Verification items for the finished model (mm, model axes). Round coordinates to 2 decimals unless told otherwise and drop trailing zeros. Order: outer loops, then holes, each group sorted by start corner. A loop starts at its lowest first (then second) coordinate and runs counter-clockwise, first axis right, second up. Notation, with made-up numbers: M 78,46 L 128,46 A21 ccw 128,62 Z; hole C 57.25,79 d4. An arc over 180 degrees is marked long. Write item = value, one per line. Start each with the question number.
from build123d import *

# Parameters (mm, degrees)
SKETCH2_W           = 70
SKETCH2_H           = 45
BOSS_EXTRUDE1_DEPTH = 1.5
SKETCH3_R           = 1.625
SKETCH3_R_2         = 6
CUT_EXTRUDE1_DEPTH  = 2.5
CUT_EXTRUDE2_DEPTH  = 2.5


with BuildPart() as part:
    # Sketch2 → Boss-Extrude1 (new body)
    with BuildSketch(Plane(origin=(0, 0, 0), x_dir=(1, 0, 0), z_dir=(0, 1, 0))):
        Rectangle(SKETCH2_W, SKETCH2_H)
    extrude(amount=BOSS_EXTRUDE1_DEPTH)

    # Sketch3 → Cut-Extrude1 (cut, through all)
    with BuildSketch(Plane(origin=(0, 1.5, 0), x_dir=(1, 0, 0), z_dir=(0, 1, 0))):
        with Locations((-31, -18.5)):
            Circle(SKETCH3_R)
        with Locations((-31, 18.5)):
            Circle(SKETCH3_R)
        with Locations((31, 18.5)):
            Circle(SKETCH3_R)
        with Locations((31, -18.5)):
            Circle(SKETCH3_R)
        with Locations((-25, 0)):
            Circle(SKETCH3_R_2)
        with Locations((25, 0)):
            Circle(SKETCH3_R_2)
    extrude(amount=-CUT_EXTRUDE1_DEPTH, mode=Mode.SUBTRACT)

    # Sketch4 → Cut-Extrude2 (cut, through all)
    with BuildSketch(Plane(origin=(0, 1.5, 0), x_dir=(1, 0, 0), z_dir=(0, 1, 0))):
        Polygon((-10.6, -18), (-10.6, -15.4), (-15.75, -10.25), (-18, -10.25), (-18, 10.25), (-15.75, 10.25), (-8, 18), (12, 18), (12, 14), (18, 8), (18, -10.6), (15.4, -10.6), (8, -18), align=None)
    extrude(amount=-CUT_EXTRUDE2_DEPTH, mode=Mode.SUBTRACT)


solid = part.part
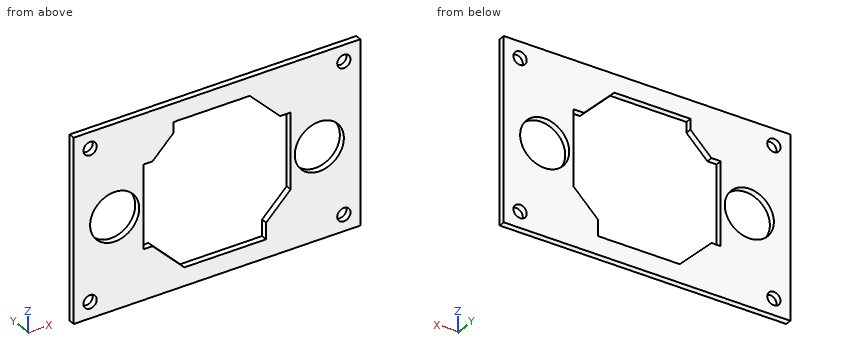
1) Scan lines: probe 1 along X at (y, z) = (0.7, 0); probe 2 along X at (y, z) = (0.3, 18.5) (3 decimals); probe 3 along Z at (x, y) = (-2, 1.35). Record each from-to range of solid material in increasing order.
2) Cross-section at A-A, the plane z = 9. Enter the section's corners in (x, y), then the cut area to 3 significant figures.
3) Cross-section at D-D, the plane y = 0.6. Enter the section's corners in (x, z) (3 decimals).
4) Cross-section at B-B, the plane x = -0.5. Enter the section's corners in (y, z).
5) Cross-section at C-C, the plane z = 0. Enter the section's corners in (x, y), then the cut area to 3 significant figures.
Geometry results:
q1.probe_1 = -35 to -31, -19 to -18, 18 to 19, 31 to 35
q1.probe_2 = -35 to -32.625, -29.375 to 29.375, 32.625 to 35
q1.probe_3 = -22.5 to -18, 18 to 22.5
q2.outline = M -35,0 L -18,0 L -18,1.5 L -35,1.5 Z; M 18,0 L 35,0 L 35,1.5 L 18,1.5 Z
q2.area = 51.0 mm^2
q3.outline = M -35,-22.5 L 35,-22.5 L 35,22.5 L -35,22.5 Z; hole C -31,-18.5 d3.25; hole C -31,18.5 d3.25; hole C -25,0 d12; hole M -18,-10.25 L -15.75,-10.25 L -8,-18 L 12,-18 L 12,-14 L 18,-8 L 18,10.6 L 15.4,10.6 L 8,18 L -10.6,18 L -10.6,15.4 L -15.75,10.25 L -18,10.25 Z; hole C 25,0 d12; hole C 31,-18.5 d3.25; hole C 31,18.5 d3.25
q4.outline = M 0,-22.5 L 1.5,-22.5 L 1.5,-18 L 0,-18 Z; M 0,18 L 1.5,18 L 1.5,22.5 L 0,22.5 Z
q5.outline = M -35,0 L -31,0 L -31,1.5 L -35,1.5 Z; M -19,0 L -18,0 L -18,1.5 L -19,1.5 Z; M 18,0 L 19,0 L 19,1.5 L 18,1.5 Z; M 31,0 L 35,0 L 35,1.5 L 31,1.5 Z
q5.area = 15.0 mm^2
